Check sheet for the modelled part. Datum: model origin and axes. Units: mm. Give positions to 0.01 mm unless a question says otherwise; leave off trailing zeros. Write each loop counter-clockwise with the first axis right and the second up, starting at its lowest first coordinate (ties: lowest second). Pieces come first, ordered by that corner, then holes.
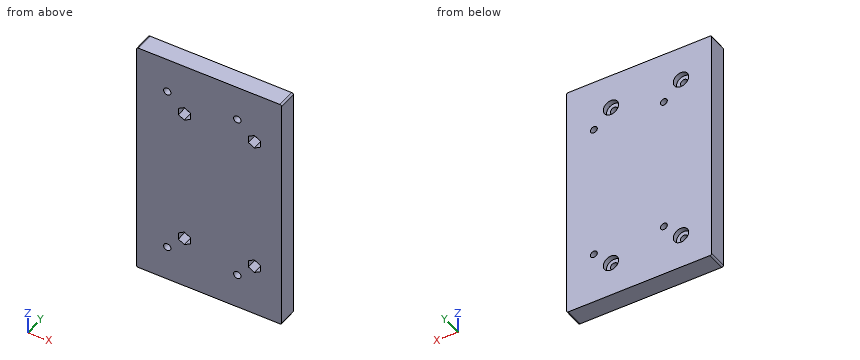
Autodesk Inventor part; units mm, degrees
ref_plane "YZ Plane" through (0, 0, 0) normal (1, 0, 0) x (0, 1, 0)
ref_plane "XZ Plane" through (0, 0, 0) normal (0, 1, 0) x (-1, 0, 0)
ref_plane "XY Plane" through (0, 0, 0) normal (0, 0, 1) x (1, 0, 0)
sketch "Esboço1" plane through (0, 0, 0) normal (0, 1, 0) x (-1, 0, 0)
  line L0 (0, 0) -> (77, 0)
  line L1 (77, 0) -> (77, -140)
  line L2 (77, -140) -> (0, -140)
  line L3 (0, -140) -> (0, 0)
  circle A0 centre (67, -20) radius 2.15
  circle A1 centre (67, -120) radius 2.15
  circle A2 centre (26, -20) radius 2.15
  circle A3 centre (26, -120) radius 2.15
  dimension "d0" = 77
  dimension "d1" = 140
  dimension "d2" = 4.3
  dimension "d3" = 4.3
  dimension "d4" = 4.3
  dimension "d5" = 4.3
  dimension "d6" = 10
  dimension "d7" = 10
  dimension "d8" = 20
  dimension "d9" = 20
  dimension "d10" = 20
  dimension "d11" = 20
  dimension "d12" = 26
  dimension "d13" = 26
extrude "Extrusão1" add sketch "Esboço1" along normal blind 11
sketch "Esboço2" plane through (0, 11, 0) normal (0, 1, 0) x (1, 0, 0)
  circle A0 centre (-67, 20) radius 2.15
  circle A1 centre (-26, 20) radius 2.15
  circle A2 centre (-26, 120) radius 2.15
  circle A3 centre (-67, 120) radius 2.15
  circle A4 centre (-67, 20) radius 4.5
  circle A5 centre (-67, 120) radius 2.15
  circle A6 centre (-67, 120) radius 4.5
  circle A7 centre (-26, 120) radius 2.15
  circle A8 centre (-26, 120) radius 4.5
  circle A9 centre (-26, 20) radius 2.15
  circle A10 centre (-26, 20) radius 4.5
  point P0 (0, 0)
  dimension "d16" = 9
  dimension "d17" = 9
  dimension "d18" = 9
  dimension "d19" = 9
extrude "Extrusão2" cut sketch "Esboço2" against normal blind 3 contours A3 | A4 | A6 | A8 | A10
sketch "Esboço3" plane through (0, 11, 0) normal (0, 1, 0) x (1, 0, 0)
  point P0 (0, 0)
sketch "Esboço4" plane through (0, 11, 0) normal (0, 1, 0) x (1, 0, 0)
  circle A0 centre (-57, 30) radius 2
  circle A1 centre (-57, 110) radius 2
  circle A2 centre (-67, 20) radius 2.15
  circle A3 centre (-67, 120) radius 2.15
  circle A4 centre (-16, 30) radius 2
  circle A5 centre (-16, 110) radius 2
  circle A6 centre (-26, 20) radius 2.15
  circle A7 centre (-26, 120) radius 2.15
  point P0 (0, 0)
  dimension "d22" = 4
  dimension "d23" = 4
  dimension "d24" = 10
  dimension "d25" = 10
  dimension "d26" = 10
  dimension "d27" = 10
  dimension "d28" = 4
  dimension "d29" = 4
  dimension "d30" = 10
  dimension "d31" = 10
  dimension "d32" = 10
  dimension "d33" = 10
extrude "Extrusão3" cut sketch "Esboço4" against normal blind 12 contours A0 | A1 | A4 | A5
sketch "Esboço5" plane through (0, 0, 0) normal (0, -1, 0) x (1, 0, 0)
  circle A0 centre (-57, -110) radius 2
  circle A1 centre (-16, -110) radius 2
  circle A2 centre (-16, -30) radius 2
  circle A3 centre (-57, -30) radius 2
  line L0 (-53.525, -112.0063) -> (-57, -114.0126)
  line L1 (-57, -114.0126) -> (-60.475, -112.0063)
  line L2 (-60.475, -112.0063) -> (-60.475, -107.9937)
  line L3 (-60.475, -107.9937) -> (-57, -105.9874)
  line L4 (-57, -105.9874) -> (-53.525, -107.9937)
  line L5 (-53.525, -107.9937) -> (-53.525, -112.0063)
  line L6 (-53.525, -32.0063) -> (-57, -34.0126)
  line L7 (-57, -34.0126) -> (-60.475, -32.0063)
  line L8 (-60.475, -32.0063) -> (-60.475, -27.9937)
  line L9 (-60.475, -27.9937) -> (-57, -25.9874)
  line L10 (-57, -25.9874) -> (-53.525, -27.9937)
  line L11 (-53.525, -27.9937) -> (-53.525, -32.0063)
  line L12 (-16, -105.9874) -> (-12.525, -107.9937)
  line L13 (-12.525, -107.9937) -> (-12.525, -112.0063)
  line L14 (-12.525, -112.0063) -> (-16, -114.0126)
  line L15 (-16, -114.0126) -> (-19.475, -112.0063)
  line L16 (-19.475, -112.0063) -> (-19.475, -107.9937)
  line L17 (-19.475, -107.9937) -> (-16, -105.9874)
  circle A4 centre (-16, -30) radius 2
  line L18 (-12.525, -32.0063) -> (-16, -34.0126)
  line L19 (-16, -34.0126) -> (-19.475, -32.0063)
  line L20 (-19.475, -32.0063) -> (-19.475, -27.9937)
  line L21 (-19.475, -27.9937) -> (-16, -25.9874)
  line L22 (-16, -25.9874) -> (-12.525, -27.9937)
  line L23 (-12.525, -27.9937) -> (-12.525, -32.0063)
  line L24 (-77, -140) -> (-77, 0)
  line L25 (0, 0) -> (0, -140)
  dimension "d36" = 6.95
  dimension "d37" = 6.95
  dimension "d38" = 6.95
  dimension "d39" = 6.95
extrude "Extrusão4" cut sketch "Esboço5" against normal blind 6 contours A0 | L0 L1 L2 L3 L4 L5 | L6 L7 L8 L9 L10 L11 | L12 L13 L14 L15 L16 L17 | L18 L19 L20 L21 L22 L23
sketch "Esboço6" plane through (-77, 0, 0) normal (0, 0, 1) x (1, 0, 0)
  line L0 (0, 0) -> (77, 0)
  line L1 (77, 0) -> (77, 11)
  line L2 (0, 11) -> (77, 11)
  line L3 (0, 0) -> (0, 11)
extrude "Extrusão5" add sketch "Esboço6" along normal blind 0.5
sketch "Esboço7" plane through (0, 0, -140) normal (0, 0, -1) x (-1, 0, 0)
  line L0 (0, 0) -> (77, 0)
  line L1 (77, 0) -> (77, 11)
  line L2 (0, 11) -> (77, 11)
  line L3 (0, 0) -> (0, 11)
  point P0 (0, 0)
extrude "Extrusão6" add sketch "Esboço7" along normal blind 0.5
sketch "Esboço8" plane through (-77, 0, 0.5) normal (-1, 0, 0) x (0, 0, 1)
  line L0 (0, 0) -> (-141, 0)
  line L1 (0, 11) -> (0, 0)
  line L2 (0, 11) -> (-141, 11)
  line L3 (-141, 0) -> (-141, 11)
  point P0 (-0.5, 0)
extrude "Extrusão7" add sketch "Esboço8" along normal blind 8
fillet "Arredondamento1" radius 1 4 edges at (-85, 5.5, 0.5) (0, 5.5, 0.5) (-85, 5.5, -140.5) (0, 5.5, -140.5)
equation "\"d4\" = d3"
equation "\"d5\" = d3"
equation "\"d7\" = d6"
equation "\"d9\" = d8"
equation "\"d10\" = d9"
equation "\"d11\" = d8"
equation "\"d16\" = d19"
equation "\"d26\" = d25"
equation "\"d27\" = d26"
equation "\"d30\" = d24"
equation "\"d33\" = d32"
equation "\"d36\" = d39"
equation "\"d37\" = d39"
equation "\"d38\" = d39"
properties part number "suporte-fonte2_TIPO2"
1) Sectioned sample at C-C on y = 3.75. Give the number of separate pieces and of enclosed holes in the cut face, then the cut area to 3 significant figures.
2) Scan lines: L1, parallel to Z at x = -26, y = 6; L2, parallel to X at y = 8.95, z = -30; L3, parallel to X at y = 9.85, z = -20. Record each from-to range of solid material in increasing order.
3) Gauge pin test, flat ends, axial feed: pin 1 (3.5 mm diameter, centred on x = -57, z = -110, fed in from +Y); pin 2 (4.5 mm diameter, centred on y = 2, z = -29.5, fed in from +X); pin 3 (5 mm diameter, centred on x = -26, z = -120, fed in from +Y); pin 4 (6.5 mm diameter, centred on x = -16, z = -30, fed in from -Y). Record the tip position at first contact, or that the pin passes through.
4) Sectioned sample at A-A on z = -120. Record the boundary of the cut face in (x, y).
5) Sectioned sample at B-B on x = -67. Record the boundary of the cut face in (y, z), then the cut area to 3 significant figures.
Answers below:
1. separate pieces: 1
1. enclosed holes: 8
1. area: 11,800 mm2
2. L1: z = -140.5 to -122.15, -117.85 to -22.15, -17.85 to 0.5
2. L2: x = -85 to -59, -55 to -18, -14 to 0
2. L3: x = -85 to -71.5, -62.5 to -30.5, -21.5 to 0
3. pin 1: passes through
3. pin 2: stops at x = 0
3. pin 3: stops at y = 8
3. pin 4: stops at y = 6
4. outline: (-85, 0) - (-69.15, 0) - (-69.15, 8) - (-71.5, 8) - (-71.5, 11) - (-85, 11) - close; (-64.85, 0) - (-28.15, 0) - (-28.15, 8) - (-30.5, 8) - (-30.5, 11) - (-62.5, 11) - (-62.5, 8) - (-64.85, 8) - close; (-23.85, 0) - (0, 0) - (0, 11) - (-21.5, 11) - (-21.5, 8) - (-23.85, 8) - close
5. outline: (0, -140.5) - (11, -140.5) - (11, -124.5) - (8, -124.5) - (8, -122.15) - (0, -122.15) - close; (0, -117.85) - (8, -117.85) - (8, -115.5) - (11, -115.5) - (11, -24.5) - (8, -24.5) - (8, -22.15) - (0, -22.15) - close; (0, -17.85) - (8, -17.85) - (8, -15.5) - (11, -15.5) - (11, 0.5) - (0, 0.5) - close
5. area: 1,430 mm2
